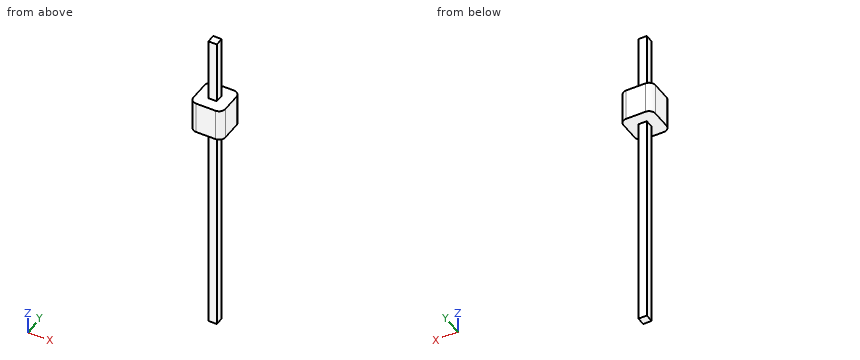
from build123d import *

# Parameters (mm, degrees)
SKETCH_1_W      = 2.54
SKETCH_1_H      = 2.54
EXTRUDE_1_DEPTH = 2.54
SKETCH_2_W      = 0.67
SKETCH_2_H      = 0.67
FILLET_1_R      = 0.5


with BuildPart() as part:
    # 草图1 → 拉伸1 (new body)
    with BuildSketch(Plane.XY):
        with Locations((0, -1.289090726)):
            Rectangle(SKETCH_1_W, SKETCH_1_H)
    extrude(amount=EXTRUDE_1_DEPTH)

    # 扫描1: sweep along a path in 草图3
    with BuildLine(Plane(origin=(0, 0, 0), x_dir=(0, 0, -1), z_dir=(1, 0, 0))) as sweep_1_path:
        Line((17.38, -1.299090726), (-7.62, -1.299090726))
    # 草图2 → 扫描1 (sweep)
    with BuildSketch(Plane(origin=(0, 0, 7.62), x_dir=(-1, 0, 0), z_dir=(0, 0, -1))):
        with Locations((0, -1.289090726)):
            Rectangle(SKETCH_2_W, SKETCH_2_H)
    sweep(path=sweep_1_path.line)

    # 圆角1
    fillet_1_edges = [part.edges().sort_by_distance(p)[0] for p in [
        (-1.27, -0.019090726, 1.27),
        (1.27, -0.019090726, 1.27),
        (1.27, -2.559090726, 1.27),
        (-1.27, -2.559090726, 1.27),
    ]]
    fillet(fillet_1_edges, radius=FILLET_1_R)


solid = part.part
Source: CAD feature listing. Evaluate the final solid. Frame: model axes, mm. Coordinates: 2 decimals unless noted, no trailing zeros. Loops run counter-clockwise (first coordinate to the right, second up) from the corner with the lowest first, then second, coordinate; pieces in that order, holes last. Notation, with made-up numbers: (-22, 8) - (-12, 8) arc R23 cw to (-12, 37) - close; hole circle Ø9 at (62.25, -9.5). An arc over 180 degrees is marked (long way). One line per question, with ' | ' between items.
1) First-contact query: P1, Ø0.7, axis at y = -1, z = -9, coming from the -X side (3 decimals); P2, Ø0.5, axis at x = 0, z = -5.5, coming from the +Y side. Flat tips, straight axial feed; report the tip coordinate or a pass-through.
Report:
P1: stops at x = -0.335 | P2: stops at y = -0.95
2) Section C-C, the plane z = 0.5. Return loops of the section in (x, y), then the cut area to 3 significant figures.
Report:
outline: (-1.27, -2.06) arc R0.5 ccw to (-0.77, -2.56) - (0.77, -2.56) arc R0.5 ccw to (1.27, -2.06) - (1.27, -0.52) arc R0.5 ccw to (0.77, -0.02) - (-0.77, -0.02) arc R0.5 ccw to (-1.27, -0.52) - close | area: 6.24 mm²
3) Section D-D, the plane z = -4.5. Return loops of the section in (x, y) (3 decimals), then the cut area to 3 significant figures.
Report:
outline: (-0.335, -1.624) - (0.335, -1.624) - (0.335, -0.954) - (-0.335, -0.954) - close | area: 0.449 mm²
4) Section B-B, the plane x = -0.1. Return loops of the section in (y, z).
Report:
outline: (-2.56, 0) - (-1.62, 0) - (-1.62, -17.38) - (-0.95, -17.38) - (-0.95, 0) - (-0.02, 0) - (-0.02, 2.54) - (-0.95, 2.54) - (-0.95, 7.62) - (-1.62, 7.62) - (-1.62, 2.54) - (-2.56, 2.54) - close
5) Section A-A, the plane y = -1.2. Return loops of the section in (x, z) (3 decimals).
Report:
outline: (-1.27, 0) - (-0.335, 0) - (-0.335, -17.38) - (0.335, -17.38) - (0.335, 0) - (1.27, 0) - (1.27, 2.54) - (0.335, 2.54) - (0.335, 7.62) - (-0.335, 7.62) - (-0.335, 2.54) - (-1.27, 2.54) - close
6) Line query: line 1 along Z through (x, y) = (0.6, -1.7); line 2 along X through (y, z) = (-1.5, -14) (3 decimals); line 3 along Y through (x, z) = (0.15, 3.25). Output: solid intervals per line, ascending.
Report:
line 1: z = 0 to 2.54 | line 2: x = -0.335 to 0.335 | line 3: y = -1.62 to -0.95
